```python
from build123d import *

# Parameters (mm, degrees)
SKETCH_1_R             = 1.5
SKETCH_1_R_2           = 17.5
SM_BASE_FLANGE_1_DEPTH = 2
FILLET_1_R             = 20


# Sheet-metal steps are written as plain solids
with BuildPart() as part:
    # Sketch 1 → 基体-法兰1 (new body)
    with BuildSketch(Plane.XY):
        with BuildLine():
            Line((22.555487137, 4.5), (75, 4.5))
            Line((75, 4.5), (75, -4.5))
            Line((75, -4.5), (22.555487137, -4.5))
            ThreePointArc((22.555487137, -4.5), (0, -23), (-22.555487137, -4.5))
            Line((-22.555487137, -4.5), (-75, -4.5))
            Line((-75, -4.5), (-75, 4.5))
            Line((-75, 4.5), (-22.555487137, 4.5))
            ThreePointArc((-22.555487137, 4.5), (0, 23), (22.555487137, 4.5))
        make_face()
        with Locations((0, 20.75)):
            Circle(SKETCH_1_R, mode=Mode.SUBTRACT)
        with Locations((14.67246571, 14.67246571)):
            Circle(SKETCH_1_R, mode=Mode.SUBTRACT)
        with Locations((14.67246571, -14.67246571)):
            Circle(SKETCH_1_R, mode=Mode.SUBTRACT)
        with Locations((0, -20.75)):
            Circle(SKETCH_1_R, mode=Mode.SUBTRACT)
        with Locations((-14.67246571, -14.67246571)):
            Circle(SKETCH_1_R, mode=Mode.SUBTRACT)
        with Locations((-14.67246571, 14.67246571)):
            Circle(SKETCH_1_R, mode=Mode.SUBTRACT)
        Circle(SKETCH_1_R_2, mode=Mode.SUBTRACT)
        with Locations((-70, 0)):
            Circle(SKETCH_1_R, mode=Mode.SUBTRACT)
        with Locations((-50, 0)):
            Circle(SKETCH_1_R, mode=Mode.SUBTRACT)
        with Locations((-30, 0)):
            Circle(SKETCH_1_R, mode=Mode.SUBTRACT)
        with Locations((30, 0)):
            Circle(SKETCH_1_R, mode=Mode.SUBTRACT)
        with Locations((50, 0)):
            Circle(SKETCH_1_R, mode=Mode.SUBTRACT)
        with Locations((70, 0)):
            Circle(SKETCH_1_R, mode=Mode.SUBTRACT)
    extrude(amount=-SM_BASE_FLANGE_1_DEPTH)

    # 圆角1
    fillet_1_edges = [part.edges().sort_by_distance(p)[0] for p in [
        (22.555487137, -4.5, -1),
        (-22.555487137, -4.5, -1),
        (-22.555487137, 4.5, -1),
        (22.555487137, 4.5, -1),
    ]]
    fillet(fillet_1_edges, radius=FILLET_1_R)


solid = part.part
```
Input: part model. Units: mm. Frame: model coordinates. Round coordinates to 2 decimals unless told otherwise and drop trailing zeros. Write each loop counter-clockwise with the first axis right and the second up, starting at its lowest first coordinate (ties: lowest second). Pieces come first, ordered by that corner, then holes. Notation, with made-up numbers: (44.5, 53.5) - (70.5, 53.5) arc R33 ccw to (70.5, 92.5) - close; hole circle Ø10 at (34.25, -0.5). An arc over 180 degrees is marked (long way). Write item = value, one per line.
(1) Section query C-C on x = -50. Output: boundary loops of the cut face in (y, z).
Geometry check:
outline = (-4.5, -2) - (-1.5, -2) - (-1.5, 0) - (-4.5, 0) - close; (1.5, -2) - (4.5, -2) - (4.5, 0) - (1.5, 0) - close
(2) Section query B-B on y = -11. Output: boundary loops of the cut face in (x, z), then the cut area to 3 significant figures.
Geometry check:
outline = (-20.58, -2) - (-13.61, -2) - (-13.61, 0) - (-20.58, 0) - close; (13.61, -2) - (20.58, -2) - (20.58, 0) - (13.61, 0) - close
area = 27.9 mm^2
(3) Material intervals for probe 1 along Y at (x, z) = (0, -0.65); probe 2 along X at (y, z) = (-15, -0.3); probe 3 along X at (y, z) = (-16, -0.1), sorted ascending.
Geometry check:
probe_1 = -23 to -22.25, -19.25 to -17.5, 17.5 to 19.25, 22.25 to 23
probe_2 = -17.44 to -16.14, -13.21 to -9.01, 9.01 to 13.21, 16.14 to 17.44
probe_3 = -16.52 to -15.37, -13.97 to -7.09, 7.09 to 13.97, 15.37 to 16.52
(4) Pull-direction query (X, two-part tool) for faces 1 (the cylindrical face through (-31.5, 0.07, -0.99)), 2 (the cylindrical face through (-25.942, -6.844, -1.014)), 3 (the flat face through (17, -5, 0)), 4 (the cylindrical face through (0, -23, -1)); classes: +X half, -X half, draft (parallel to the pull), parting line (faces both ways), or undercut.
Geometry check:
face_1 = undercut
face_2 = -X half
face_3 = draft
face_4 = parting line
(5) Section query D-D on y = 0. State how many separate pieces and enclosed holes the cut face has, then the cut area to 3 significant figures.
Geometry check:
separate_pieces = 8
enclosed_holes = 0
area = 194 mm^2
(6) Contact query for flat-ended pins moving along their axis: pin 1 Ø5 at (x, y) = (14.67, -14.67) entering from -Z; pin 2 Ø1 at (x, z) = (-50, -1) entering from -Y. Output: stop coordinate, or through.
Geometry check:
pin_1 = -2
pin_2 = -4.5
(7) Section query A-A on x = 0. Output: boundary loops of the cut face in (y, z), then the cut area to 3 significant figures.
Geometry check:
outline = (-23, -2) - (-22.25, -2) - (-22.25, 0) - (-23, 0) - close; (-19.25, -2) - (-17.5, -2) - (-17.5, 0) - (-19.25, 0) - close; (17.5, -2) - (19.25, -2) - (19.25, 0) - (17.5, 0) - close; (22.25, -2) - (23, -2) - (23, 0) - (22.25, 0) - close
area = 10.0 mm^2
